from build123d import *

# Parameters (mm, degrees)
SKETCH_1_R          = 57.5
EXTRUDE_1_DEPTH     = 5
SKETCH_2_R          = 57.5
SKETCH_2_R_2        = 52.5
EXTRUDE_2_DEPTH     = 30
SKETCH_3_R          = 1.65
SKETCH_3_W          = 55
SKETCH_3_H          = 60
CUT_EXTRUDE_1_DEPTH = 87.674679117
CUT_EXTRUDE_START   = -30
CUT_EXTRUDE_2_DEPTH = 30
CHAMFER_1_SIZE      = 2


with BuildPart() as part:
    # ｽｹｯﾁ1 → ﾎﾞｽ - 押し出し1 (new body)
    with BuildSketch(Plane(origin=(0, 0, 0), x_dir=(0, 0, -1), z_dir=(1, 0, 0))):
        Circle(SKETCH_1_R)
    extrude(amount=EXTRUDE_1_DEPTH)

    # ｽｹｯﾁ2 → ﾎﾞｽ - 押し出し2 (add)
    with BuildSketch(Plane(origin=(5, 0, 0), x_dir=(0, 0, -1), z_dir=(1, 0, 0))):
        Circle(SKETCH_2_R)
        Circle(SKETCH_2_R_2, mode=Mode.SUBTRACT)
    extrude(amount=EXTRUDE_2_DEPTH)

    # ｽｹｯﾁ3 → ｶｯﾄ - 押し出し1 (cut, through all)
    with BuildSketch(Plane(origin=(5, 0, 0), x_dir=(0, 0, -1), z_dir=(1, 0, 0))):
        with Locations((-22.25, 20)):
            Circle(SKETCH_3_R)
        with Locations(Location((-22.25, -20, 0), (0, 0, 180))):
            Circle(SKETCH_3_R)
        with Locations(Location((42.25, 20, 0), (0, 0, 180))):
            Circle(SKETCH_3_R)
        with Locations((42.25, -20)):
            Circle(SKETCH_3_R)
        with Locations((10, 0)):
            Rectangle(SKETCH_3_W, SKETCH_3_H)
    extrude(amount=-CUT_EXTRUDE_1_DEPTH, mode=Mode.SUBTRACT)

    # ｽｹｯﾁ4 → ｶｯﾄ - 押し出し2 (cut)
    with BuildSketch(Plane(origin=(35, 0, 0), x_dir=(0, 0, -1), z_dir=(1, 0, 0)).offset(CUT_EXTRUDE_START)):
        with BuildLine():
            ThreePointArc((20, 53.909646632), (0, 57.5), (-20, 53.909646632))
            Line((-20, 53.909646632), (-20, 48.541219597))
            ThreePointArc((-20, 48.541219597), (0, 52.5), (20, 48.541219597))
            Line((20, 48.541219597), (20, 53.909646632))
        make_face()
        with BuildLine():
            Line((-48.541219597, 20), (-53.909646632, 20))
            ThreePointArc((-53.909646632, 20), (-57.5, 0), (-53.909646632, -20))
            Line((-53.909646632, -20), (-48.541219597, -20))
            ThreePointArc((-48.541219597, -20), (-52.5, 0), (-48.541219597, 20))
        make_face()
        with BuildLine():
            Line((53.909646632, 20), (48.541219597, 20))
            ThreePointArc((48.541219597, 20), (52.5, 0), (48.541219597, -20))
            Line((48.541219597, -20), (53.909646632, -20))
            ThreePointArc((53.909646632, -20), (57.5, 0), (53.909646632, 20))
        make_face()
        with BuildLine():
            Line((-20, -48.541219597), (-20, -53.909646632))
            ThreePointArc((-20, -53.909646632), (0, -57.5), (20, -53.909646632))
            Line((20, -53.909646632), (20, -48.541219597))
            ThreePointArc((20, -48.541219597), (0, -52.5), (-20, -48.541219597))
        make_face()
    extrude(amount=CUT_EXTRUDE_2_DEPTH, mode=Mode.SUBTRACT)

    # 面取り1
    chamfer_1_edges = [part.edges().sort_by_distance(p)[0] for p in [
        (0, 0, 57.5),
    ]]
    chamfer(chamfer_1_edges, length=CHAMFER_1_SIZE)


solid = part.part
Design review of the part built by this model. Coordinates are the model's own, in mm. A direction names the side the tool comes from. Coordinates: 2 decimals unless noted, no trailing zeros. Loops run counter-clockwise (first coordinate to the right, second up) from the corner with the lowest first, then second, coordinate; pieces in that order, holes last.
Item 1: Wall thickness on L1, parallel to Y at x = 1.4, z = 22.25; L2, parallel to Y at x = 2, z = -42; L3, parallel to X at y = -38.5, z = -8: over which ranges is each line inside the solid? List them lowest first.
Completed:
L1: y = -52.37 to -21.65, -18.35 to 18.35, 21.65 to 52.37
L2: y = -39.27 to -21.63, -18.37 to 18.37, 21.63 to 39.27
L3: x = 0 to 5
Item 2: For faces 1 (the flat face through (3, 0, -37.5)), 2 (the flat face through (20, -51, 20)), 3 (the flat face through (20, 20, 51)), 4 (the cylindrical face through (19.79, -36.917, 37.328)), list the 3-axis set-ups (+Z, -Z, +X, -X, +Y, -Y) from which the entire face can be reached by the end or side of a thin tool; tool diameter is ignored.
Completed:
face 1: +X, -X
face 2: +X, +Y, -Y
face 3: +Z, -Z, +X
face 4: +X
Item 3: Add section B-B (z = 0). Write out the cut boundary in (x, y), and give its area (3 significant figures).
Completed:
outline: (0, -55.5) - (2, -57.5) - (5, -57.5) - (5, -30) - (0, -30) - close; (0, 30) - (5, 30) - (5, 57.5) - (2, 57.5) - (0, 55.5) - close
area: 271 mm2
Item 4: Clearance check with flat-ended pins moving along their axes: pin 1 (4.5 mm diameter, centred on x = 26, y = -51, fed in from -Z); pin 2 (4.5 mm diameter, centred on x = 22.5, z = -51, fed in from -Y); pin 3 (6 mm diameter, centred on y = 10, z = -41.5, fed in from +X). State where each tip first meets the part, or that it passes through.
Completed:
pin 1: stops at z = -30.49
pin 2: stops at y = -30.49
pin 3: stops at x = 5
Item 5: Add section A-A (y = 0). Write out the cut boundary in (x, z), and give its area (3 significant figures).
Completed:
outline: (0, -55.5) - (2, -57.5) - (5, -57.5) - (5, -37.5) - (0, -37.5) - close; (0, 17.5) - (5, 17.5) - (5, 57.5) - (2, 57.5) - (0, 55.5) - close
area: 296 mm2
Item 6: Draft analysis for pull direction Z (two halves, no side actions). For faces 5 (the cylindrical face through (18.269, -22.023, -53.115)), 6 (the flat face through (20, -20, -51)), 7 (the cylindrical face through (19.79, 37.328, 36.917)), state which applies: pulls with the +Z half, pulls with the -Z half, needs draft (parallel to the pull), parting line crosses it, or undercut.
Completed:
face 5: parting line crosses it
face 6: needs draft
face 7: undercut
Item 7: Add section C-C (x = 13.5). Write out the cut boundary in (y, z), and give its area (3 significant figures).
Completed:
outline: (-53.91, -20) arc R57.5 ccw to (-20, -53.91) - (-20, -48.54) arc R52.5 cw to (-48.54, -20) - close; (-53.91, 20) - (-48.54, 20) arc R52.5 cw to (-20, 48.54) - (-20, 53.91) arc R57.5 ccw to start; (20, -53.91) arc R57.5 ccw to (53.91, -20) - (48.54, -20) arc R52.5 cw to (20, -48.54) - close; (20, 48.54) arc R52.5 cw to (48.54, 20) - (53.91, 20) arc R57.5 ccw to (20, 53.91) - close
area: 909 mm2
Item 8: Add section D-D (z = 22.25). Give the number of separate pieces and of enclosed holes in the cut face, and give its area (3 significant figures).
Completed:
separate pieces: 3
enclosed holes: 0
area: 821 mm2
